Autodesk Inventor part; units mm, degrees
ref_plane "YZ Plane" through (0, 0, 0) normal (1, 0, 0) x (0, 1, 0)
ref_plane "XZ Plane" through (0, 0, 0) normal (0, 1, 0) x (-1, 0, 0)
ref_plane "XY Plane" through (0, 0, 0) normal (0, 0, 1) x (1, 0, 0)
sketch "Sketch1" plane through (0, 0, 0) normal (0, 1, 0) x (-1, 0, 0)
  line L0 (0, 0) -> (9.525, 0)
  line L1 (9.525, 0) -> (9.525, -114.3)
  line L2 (9.525, -114.3) -> (0, -114.3)
  line L3 (0, -114.3) -> (0, 0)
  dimension "d0" = 9.525
  dimension "d1" = 114.3
extrude "Extrusion1" add sketch "Sketch1" along normal blind 9.525
sketch "Sketch2" plane through (0, 9.525, 0) normal (0, 1, 0) x (1, 0, 0)
  point P0 (0, 0)
  point P1 (-2.3813, 12.7)
sketch "Sketch3" plane through (0, 9.525, 0) normal (0, 1, 0) x (1, 0, 0)
  line L0 (-2.3876, 12.7) -> (-7.1501, 12.7)
  line L1 (-7.1501, 12.7) -> (-7.1501, 101.6)
  line L2 (-7.1501, 101.6) -> (-2.3876, 101.6)
  line L3 (-2.3876, 101.6) -> (-2.3876, 12.7)
  point P0 (0, 0)
  dimension "d4" = 4.7625
  dimension "d5" = 88.9
extrude "Extrusion2" cut sketch "Sketch3" against normal blind 9.525
sketch "Sketch4" plane through (0, 0, 0) normal (1, 0, 0) x (0, 0, -1)
  circle A0 centre (6.1453, 4.7625) radius 3.175
  circle A1 centre (6.1453, 4.7625) radius 3.302
  point P0 (0, 0)
  dimension "d8" = 6.35
  dimension "d9" = 6.604
extrude "Extrusion3" cut sketch "Sketch4" against normal blind 8.255 contours A0 | A1
sketch "Sketch5" plane through (0, 0, 0) normal (1, 0, 0) x (0, 0, -1)
  point P0 (0, 0)
  point P1 (107.95, 4.7625)
sketch "Sketch6" plane through (0, 0, 0) normal (1, 0, 0) x (0, 0, -1)
  circle A0 centre (6.1453, 4.7625) radius 3.302
  circle A1 centre (6.1453, 4.7625) radius 3.302
  point P0 (0, 0)
extrude "Extrusion4" add sketch "Sketch6" against normal blind 9.2075
sketch "Sketch7" plane through (0, 0, 0) normal (1, 0, 0) x (0, 0, -1)
  circle A0 centre (4.7752, 4.7625) radius 3.302
  circle A1 centre (109.5248, 4.7752) radius 3.302
  point P0 (0, 0)
  dimension "d14" = 6.604
  dimension "d15" = 6.604
extrude "Extrusion5" cut sketch "Sketch7" against normal blind 7.62
sketch "Sketch8" plane through (-9.525, 0, -114.3) normal (-1, 0, 0) x (0, 0, 1)
  line L0 (61.9125, 3.175) -> (52.3875, 3.175)
  line L1 (52.3875, 3.175) -> (52.3875, 6.35)
  line L2 (52.3875, 6.35) -> (61.9125, 6.35)
  line L3 (61.9125, 6.35) -> (61.9125, 3.175)
  line L4 (61.9125, 3.175) -> (52.3875, 6.35) construction
  line L5 (52.3875, 3.175) -> (61.9125, 6.35) construction
  point P0 (114.3, 0)
  point P1 (57.15, 4.7625)
  dimension "d18" = 9.525
  dimension "d19" = 3.175
extrude "Extrusion6" add sketch "Sketch8" along normal blind 19.05
sketch "Sketch9" plane through (-9.525, 6.35, -52.3875) normal (0, 1, 0) x (1, 0, 0)
  point P0 (9.525, -52.3875)
sketch "Sketch10" plane through (-28.575, 0, -114.3) normal (-1, 0, 0) x (0, 0, 1)
  point P0 (114.3, 0)
sketch "Sketch11" plane through (-28.575, 0, -114.3) normal (-1, 0, 0) x (0, 0, 1)
  line L0 (61.9125, 3.175) -> (52.3875, 3.175)
  line L1 (52.3875, 6.35) -> (61.9125, 6.35)
  line L2 (52.3875, 3.175) -> (61.9125, 3.175)
  line L3 (61.9125, 3.175) -> (61.9125, 6.35)
  line L4 (61.9125, 6.35) -> (52.3875, 6.35)
  line L5 (52.3875, 6.35) -> (52.3875, 3.175)
  point P0 (114.3, 0)
extrude "Extrusion7" add sketch "Sketch11" along normal blind 6.35
sketch "Sketch12" plane through (-34.925, 0, -114.3) normal (-1, 0, 0) x (0, 0, 1)
  line L0 (52.3875, 6.35) -> (61.9125, 6.35)
  line L1 (52.3875, 3.175) -> (52.3875, 6.35)
  line L2 (61.9125, 6.35) -> (52.3875, 6.35)
  line L3 (52.3875, 6.35) -> (52.3875, 3.175)
  line L4 (52.3875, 3.175) -> (61.9125, 3.175)
  line L5 (61.9125, 3.175) -> (61.9125, 6.35)
  point P0 (114.3, 0)
sketch "Sketch13" plane through (-9.525, 3.175, -61.9125) normal (0, -1, 0) x (1, 0, 0)
  circle A0 centre (-20.6248, 4.7625) radius 3.175
  point P0 (9.525, 61.9125)
  dimension "d24" = 6.35
extrude "Extrusion8" cut sketch "Sketch13" against normal blind 6.35
fillet "Fillet1" radius 3.175 2 edges at (-9.525, 6.35, -57.15) (-9.525, 3.175, -57.15)
fillet "Fillet2" radius 3.175 2 edges at (-9.525, 4.7625, -52.3875) (-9.525, 4.7625, -61.9125)
sketch "Sketch14" plane through (-9.525, 0, 0) normal (-1, 0, 0) x (0, 0, 1)
  line L0 (-61.9125, 3.175) -> (-52.3875, 3.175)
  line L1 (-61.9125, 3.175) -> (-87.3125, 3.175)
  line L2 (-87.3125, 3.175) -> (-87.3125, 6.35)
  line L3 (-87.3125, 6.35) -> (-61.9125, 6.35)
  line L4 (-61.9125, 6.35) -> (-61.9125, 3.175)
  line L5 (-49.2125, 0) -> (-52.3875, 3.175)
  line L6 (-52.3875, 3.175) -> (-26.9875, 3.175)
  line L7 (-26.9875, 3.175) -> (-26.9875, 6.35)
  line L8 (-26.9875, 6.35) -> (-52.3875, 6.35)
  line L9 (-52.3875, 6.35) -> (-52.3875, 3.175)
  point P0 (0, 0)
  dimension "d29" = 25.4
  dimension "d30" = 25.4
sketch "Sketch15" plane through (-9.525, 0, 0) normal (-1, 0, 0) x (0, 0, 1)
  point P0 (0, 0)
sketch "Sketch16" plane through (-34.925, 6.35, -52.3875) normal (0, 1, 0) x (1, 0, 0)
  arc A0 (25.3996, 34.9251) -> (25.3996, -25.3998) centre (30.609, 4.7627) ccw
  line L0 (25.3996, 34.9251) -> (25.3996, -25.3998)
  line L1 (25.4, 61.9125) -> (25.4, 12.7)
  point P0 (34.925, -52.3875)
sketch "Sketch17" plane through (-34.925, 6.35, -52.3875) normal (0, 1, 0) x (1, 0, 0)
  circle A0 centre (4.7752, 4.7625) radius 3.175
  point P0 (34.925, -52.3875)
sketch "Sketch18" plane through (0, 9.525, 0) normal (0, 1, 0) x (1, 0, 0)
  point P0 (0, 0)
sketch "Sketch19" plane through (-9.525, 0, -114.3) normal (-1, 0, 0) x (0, 0, 1)
  point P0 (114.3, 0)
extrude "Extrusion9" add sketch "Sketch16" against normal blind 3.175
hole "Hole1" at (-30.1498, 6.35, -57.15) direction (0, -1, 0) diameter 6.35 depth 3.048 tip angle 118
sketch "Sketch20" plane through (0, 9.525, 0) normal (0, 1, 0) x (1, 0, 0)
  line L0 (-9.525, 0) -> (-9.525, 49.2125)
  line L1 (-9.525, 0) -> (-38.3402, 0)
  line L2 (-38.3402, 0) -> (-38.3402, 114.3)
  line L3 (-38.3402, 114.3) -> (-9.525, 114.3)
  line L4 (-9.525, 114.3) -> (-9.525, 0)
  point P0 (0, 0)
extrude "Extrusion10" cut sketch "Sketch20" against normal blind 25.4
sketch "Sketch21" plane through (0, 0, 0) normal (1, 0, 0) x (0, 0, -1)
  circle A0 centre (4.7752, 4.7625) radius 3.302
  circle A1 centre (4.7752, 4.7625) radius 3.302
  circle A2 centre (109.5248, 4.7752) radius 3.302
  circle A3 centre (109.5248, 4.7752) radius 3.302
  point P0 (0, 0)
extrude "Extrusion11" cut sketch "Sketch21" against normal blind 12.7
equation "\"d38\" = Thickness"
equation "\"BendRadius\" = Thickness"
equation "\"BendReliefWidth\" = Thickness"
equation "\"BendReliefDepth\" = 0.5 * Thickness"
equation "\"CornerReliefSize\" = 4 * Thickness"
equation "\"MinimumRemnant\" = 2 * Thickness"
equation "\"TransitionRadius\" = BendRadius"
equation "\"JacobiRadiusSize\" = Thickness"
equation "\"GapSize\" = Thickness"
properties part number "MTV horizantal connector (12.10)"
Could you check a few things on this model? Use its own coordinates, in mm. A direction names the side the tool comes from. Round coordinates to 2 decimals unless told otherwise and drop trailing zeros. Write each loop counter-clockwise with the first axis right and the second up, starting at its lowest first coordinate (ties: lowest second). Pieces come first, ordered by that corner, then holes. Notation, with made-up numbers: (62, 64) - (109, 64) arc R15 ccw to (109, 70) - close; hole circle Ø11 at (21.5, 22). An arc over 180 degrees is marked (long way). Put each result on its own line as item: value. Start each with the question number.
(1) Will this pin go through, and if not, where does the flat tip stop? pin 1 (4 mm diameter, centred on x = -6, y = 6, fed in from +Z).
(2) I want a section at C-C, the plane z = -7. Please give me the cut outline in (x, y) (3 decimals), plus the area to 3 significant figures.
(3) Thinking about a two-plate mould opening in Z: for faces 3 (the flat face through (-5, 5, -114.3)), 4 (the cylindrical face through (-4.696, 1.846, -111.048)), 5 (the flat face through (-9.525, 5, -56)), which applies, released by +Z, released by -Z, zero draft, split by the parting line, or undercut?
(4) I want a section at B-B, the plane x = -4. Please give me the cut outline in (y, z) (1 decimal), plus the area to 3 significant figures.
(5) For faces 1 (the flat face through (-2.388, 5, -58)), 2 (the flat face through (-2, 9.525, -56)), which set-ups out of +Z, -Z, +X, -X, +Y, -Y let a thin tool reach every point of the face, with its end or its side?
(6) I need wall thicknesses on probe 1 along X at (y, z) = (3.75, -69) (3 decimals); probe 2 along Z at (x, y) = (-8.5, 6); probe 3 along Z at (x, y) = (-2.5, 9). Which ranges of each line are inside material? Lowest first, please.
(7) I want a section at A-A, the plane z = -25. Please give me the cut outline in (x, y) (3 decimals).
Here are the results:
1. pin 1: stops at z = 0
2. outline: (-9.525, 0) - (0, 0) - (0, 2.323) - (-9.525, 2.323) - close; (-9.525, 7.202) - (0, 7.202) - (0, 9.525) - (-9.525, 9.525) - close
2. area: 44.2 mm^2
3. face 3: released by -Z
3. face 4: undercut
3. face 5: zero draft
4. outline: (0, -114.3) - (9.5, -114.3) - (9.5, -101.6) - (0, -101.6) - close; (0, -12.7) - (9.5, -12.7) - (9.5, 0) - (0, 0) - close; hole circle Ø6.6 at (4.8, -109.5); hole circle Ø6.6 at (4.8, -4.8)
4. area: 173 mm^2
5. face 1: +Y, -Y
5. face 2: +Z, -Z, +X, -X, +Y
6. probe 1: x = -9.525 to -7.15, -2.388 to 0
6. probe 2: z = -114.3 to -112.59, -106.46 to -7.84, -1.71 to 0
6. probe 3: z = -114.3 to -101.6, -12.7 to 0
7. outline: (-9.525, 0) - (-7.15, 0) - (-7.15, 9.525) - (-9.525, 9.525) - close; (-2.388, 0) - (0, 0) - (0, 9.525) - (-2.388, 9.525) - close
